Answer from the drawing. Dimensions are ordinates in mm from the lowest x, y and z of the part. A direction names the side the tool comes from. Round coordinates to 2 decimals unless told otherwise and drop trailing zeros. Write each loop counter-clockwise with the first axis right and the second up, starting at its lowest first coordinate (ties: lowest second). Pieces come first, ordered by that corner, then holes. Notation, with made-up numbers: (-35.5, -38) - (-10.5, -38) arc R36 ccw to (-10.5, 1) - close; hole circle Ø2 at (-23.75, 28.25). An arc over 180 degrees is marked (long way). Answer as CSV lines item,"result". Start each with the question number.
1) Find section C-C on x = 55. Determine the outline of the cut face in (y, z).
2) Consider line 1 along X through (y, z) = (4.15, 4.5); line 2 along X through (y, z) = (4, 195); line 3 along X through (y, z) = (8.5, 85). Determine where each line is inside the solid, lowest interval first.
3) Find section B-B on y = 29.5. Determine the outline of the cut face in (x, z).
4) Each of these flat-tipped pins is pushed along its axis until it touches: pin 1 (12 mm diameter, centred on y = 25.5, z = 139.5, fed in from -X); pin 2 (6.5 mm diameter, centred on x = 136.881, z = 4.5, fed in from +Y); pin 3 (3.5 mm diameter, centred on y = 99.7, z = 4.5, fed in from -X). Where does it stop, or does it pass through?
5) Which of the six approach directions +Z, -Z, +X, -X, +Y, -Y give full straight-line access (tool end or side, diameter ignored) to the marked faces 1 and 2?
6) Find section A-A on z = 70. Determine the outline of the cut face in (x, y), then the cut area to 3 significant figures.
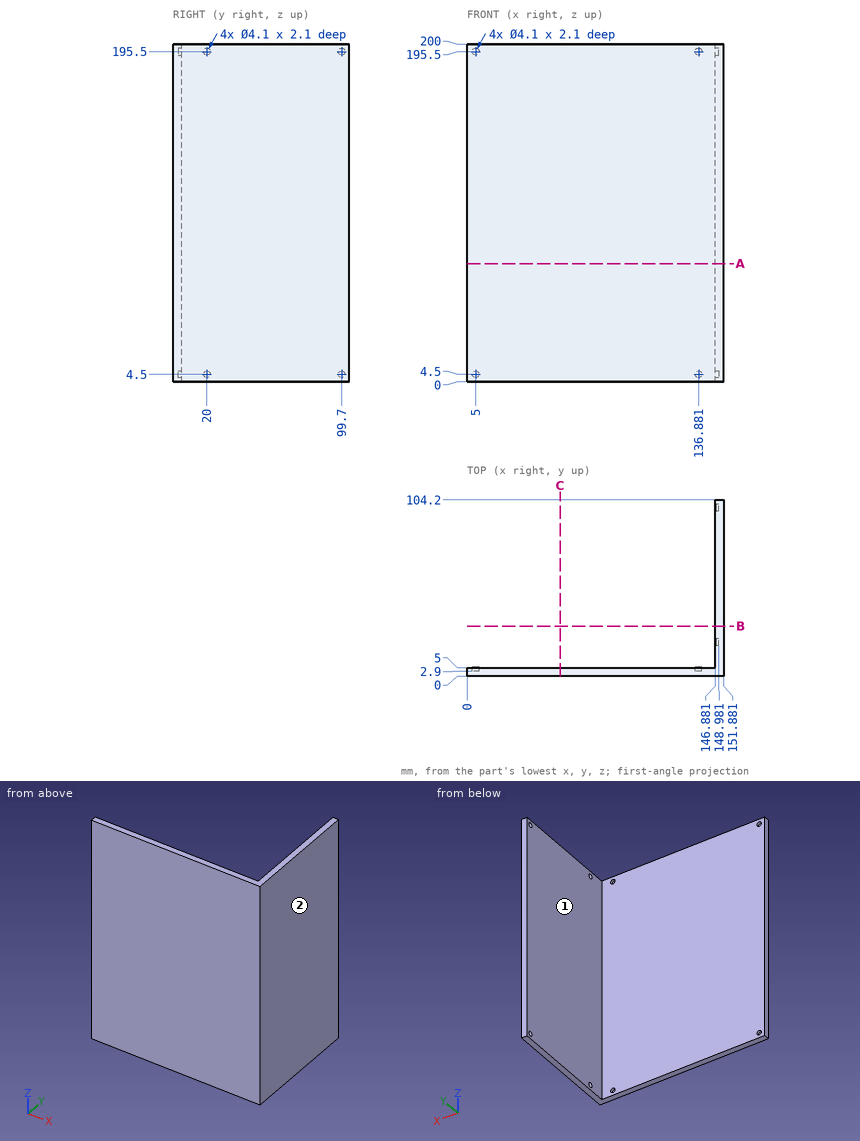
Check values:
1,outline,"(0, 0) - (5, 0) - (5, 200) - (0, 200) - close"
2,line 1,"x = 0 to 2.95, 7.05 to 134.83, 138.93 to 151.88"
2,line 2,"x = 0 to 3.01, 6.99 to 134.89, 138.87 to 151.88"
2,line 3,"x = 146.88 to 151.88"
3,outline,"(146.88, 0) - (151.88, 0) - (151.88, 200) - (146.88, 200) - close"
4,pin 1,"stops at x = 146.88"
4,pin 2,"stops at y = 5"
4,pin 3,"stops at x = 148.98"
5,face 1,"+Z, -Z, -X, +Y"
5,face 2,"+Z, -Z, +X, +Y, -Y"
6,outline,"(0, 0) - (151.88, 0) - (151.88, 104.2) - (146.88, 104.2) - (146.88, 5) - (0, 5) - close"
6,area,"1,260 mm^2"
